```python
from build123d import *

# Parameters (mm, degrees)
SKETCH1_R           = 32.75
BOSS_EXTRUDE1_DEPTH = 80.75
SKETCH12_R          = 6
BOSS_EXTRUDE5_DEPTH = 63
SKETCH14_R          = 3
CUT_EXTRUDE2_DEPTH  = 10
CIRPATTERN2_COUNT   = 4
CUT_EXTRUDE5_START  = -1.5
SKETCH17_R          = 50
CUT_EXTRUDE5_DEPTH  = 170.510044343
SHELL1_T            = -2
CHAMFER2_SIZE       = 2


with BuildPart() as part:
    # Sketch1 → Boss-Extrude1 (new, symmetric)
    with BuildSketch(Plane.XY):
        Circle(SKETCH1_R)
    extrude(amount=BOSS_EXTRUDE1_DEPTH, both=True)

    # Sketch10 → Revolve1 (revolve)
    with BuildSketch(Plane(origin=(0, 0, 0), x_dir=(0, 0, -1), z_dir=(1, 0, 0)), mode=Mode.PRIVATE) as revolve1_sk:
        Polygon((-97.75, 0), (-97.75, 14), (-80.75, 19), (-80.75, 0), align=None)
    revolve(revolve1_sk.sketch.rotate(Axis((0, 0, 1000), (0, 0, -1)), 90), axis=Axis((0, 0, 1000), (0, 0, -1)))

    # Sketch12 → Boss-Extrude5 (add)
    with BuildSketch(Plane.XY.offset(97.75)):
        Circle(SKETCH12_R)
    extrude(amount=BOSS_EXTRUDE5_DEPTH)

    # Sketch14 → Cut-Extrude2 (cut)
    with BuildSketch(Plane(origin=(0, 0, -80.75), x_dir=(-1, 0, 0), z_dir=(0, 0, -1))):
        with Locations((21, 0)):
            Circle(SKETCH14_R)
    cut_extrude2 = extrude(amount=-CUT_EXTRUDE2_DEPTH, mode=Mode.SUBTRACT)

    # CirPattern2: Cut-Extrude2 ×4 about axis
    cirpattern2_axis = Axis((0, 0, 0), (0, 0, 1))
    for i in range(1, CIRPATTERN2_COUNT):
        add(cut_extrude2.rotate(cirpattern2_axis, i * 360 / CIRPATTERN2_COUNT), mode=Mode.SUBTRACT)

    # Sketch17 → Cut-Extrude5 (cut, through all)
    with BuildSketch(Plane.XY.offset(80.75).offset(CUT_EXTRUDE5_START)):
        Circle(SKETCH17_R)
    extrude(amount=CUT_EXTRUDE5_DEPTH, mode=Mode.SUBTRACT)

    # Shell1
    shell1_openings = [part.faces().sort_by_distance(p)[0] for p in [
        (0, 0, 79.25),
    ]]
    offset(amount=SHELL1_T, openings=shell1_openings, kind=Kind.INTERSECTION)

    # Chamfer2
    chamfer2_edges = [part.edges().sort_by_distance(p)[0] for p in [
        (-30.75, 0, 79.25),
    ]]
    chamfer(chamfer2_edges, length=CHAMFER2_SIZE - 0.0001)  # a hair under: the kernel refuses the full size


solid = part.part
```
Part model, mm, in its own coordinate system. A direction names the side the tool comes from. Round coordinates to 2 decimals unless told otherwise and drop trailing zeros. Write each loop counter-clockwise with the first axis right and the second up, starting at its lowest first coordinate (ties: lowest second). Pieces come first, ordered by that corner, then holes.
Item 1: Two-plate mould, pull along X, no slides. Class faces 3 (the cylindrical face through (0, 18, -76)), 4 (the flat face through (0, 0, -80.75)), 5 (the cylindrical face through (31.238, 9.837, 0.37)): +X half, -X half, draft (parallel to the pull), parting line (faces both ways), or undercut.
Results:
face 3: undercut
face 4: draft
face 5: parting line
Item 2: Which spindle directions (+Z, -Z, +X, -X, +Y, -Y) get a long thin tool onto all of the face, cutting with end or side? Do faces 1 (the flat face through (0, -21, -70.75)), 2 (the flat face through (0, 21, -68.75)). Say none if no direction does.
Results:
face 1: -Z
face 2: +Z
Item 3: Cut at B-B, the plane z = 0. Give the cut face in (x, y), plus the area to 3 significant figures.
Results:
outline: circle Ø65.5 at (0, 0); hole circle Ø61.5 at (0, 0)
area: 399 mm2
Item 4: Probe L1, parallel to X at y = -1, z = -38; L2, parallel to Y at x = 21, z = -74. List the from-to ranges inside material, lowest first.
Results:
L1: x = -32.73 to -30.73, 30.73 to 32.73
L2: y = -25.13 to -22.46, -5 to -3, 3 to 5, 22.46 to 25.13
Item 5: Drop flat-ended pins along their axis: pin 1 Ø6.5 at (x, y) = (-0.5, -20.5) entering from -Z; pin 2 Ø5 at (x, y) = (21, 0) entering from -Z; pin 3 Ø2 at (x, z) = (-13, 7) entering from -Y; pin 4 Ø5 at (x, y) = (22, -1.5) entering from +Z. Give the stop position or say it passes through.
Results:
pin 1: stops at z = -80.75
pin 2: stops at z = -70.75
pin 3: stops at y = -30.47
pin 4: stops at z = -68.75
